```python
from build123d import *

# Parameters (mm, degrees)
F0_R     = 8
F1_DEPTH = 3.5
F2_SIZE  = 3.49999
F3_R     = 3.625
F4_R     = 1.625


# Not quite as in the source:
# - a fillet or chamfer is up to 0.001 mm smaller than in the source, because OpenCascade refuses the exact size


with BuildPart() as f1:
    # F0 (on Top) → F1 (new body)
    with BuildSketch(Plane.XY):
        Circle(F0_R)
    extrude(amount=F1_DEPTH)

    # F2 (size 3.5 in the source; OpenCascade refuses exactly that, so slightly less here)
    f2_edges = [f1.edges().sort_by_distance(p)[0] for p in [
        (-8, 0, 3.5),
    ]]
    chamfer(f2_edges, length=F2_SIZE)

    # F3 (on face) → F5 section 0
    with BuildSketch(Plane.XY.offset(3.5)):
        Circle(F3_R)
    # F4 (on Top) → F5 section 1
    with BuildSketch(Plane.XY):
        Circle(F4_R)
    loft(mode=Mode.SUBTRACT)


solid = f1.part
```
Here's how the part is built. I have some questions about the finished solid (model axes, mm). Give positions to 0.01 mm unless a question says otherwise; leave off trailing zeros. Order: outer loops, then holes, each group sorted by start corner. A loop starts at its lowest first (then second) coordinate and runs counter-clockwise, first axis right, second up. Notation, with made-up numbers: (36, 82) - (51, 82) arc R26 ccw to (51, 107) - close; hole circle Ø8 at (-40, 39). An arc over 180 degrees is marked (long way). Answer as a JSON object with one key per item and string values. Group by question number.
Item 1: If we section it at B-B on z = 2.45: Please give me the cut outline in (x, y) (3 decimals), and give its area (3 significant figures).
Item 2: Please list where these lines run through material, in increasing order: probe 1 along X at (y, z) = (-2.25, 2.4); probe 2 along X at (y, z) = (-2.25, 2.6); probe 3 along Y at (x, z) = (-1.75, 1.2).
Item 3: For P1, Ø1.5, axis at x = -6, z = 2, coming from the +Y side, with a flat end and sliding along its axis, tell me the tip position at first contact or that it passes through.
Item 4: If we section it at C-C on z = 1.1: Please give me the cut outline in (x, y).
Item 5: If we mould it in two halves opening along Y, with no side actions, what happens to faces 1 (the conical face through (-1.543, -1.183, 0.559)), 2 (the flat face through (2, 0, 0)), 3 (the conical face through (-4, -3, 3))? For each: pulls with the +Y half, pulls with the -Y half, needs draft (parallel to the pull), parting line crosses it, or undercut.
Result set:
{
 "1": {"outline": "circle Ø11.1 at (0, 0); hole circle Ø6.05 at (0, 0)", "area": "68.0 mm²"},
 "2": {"probe 1": "-5.13 to -1.98, 1.98 to 5.13", "probe 2": "-4.91 to -2.15, 2.15 to 4.91", "probe 3": "-6.57 to -1.51, 1.51 to 6.57"},
 "3": {"P1": "y = 3.57"},
 "4": {"outline": "circle Ø13.8 at (0, 0); hole circle Ø4.51 at (0, 0)"},
 "5": {"face 1": "undercut", "face 2": "needs draft", "face 3": "parting line crosses it"}
}
